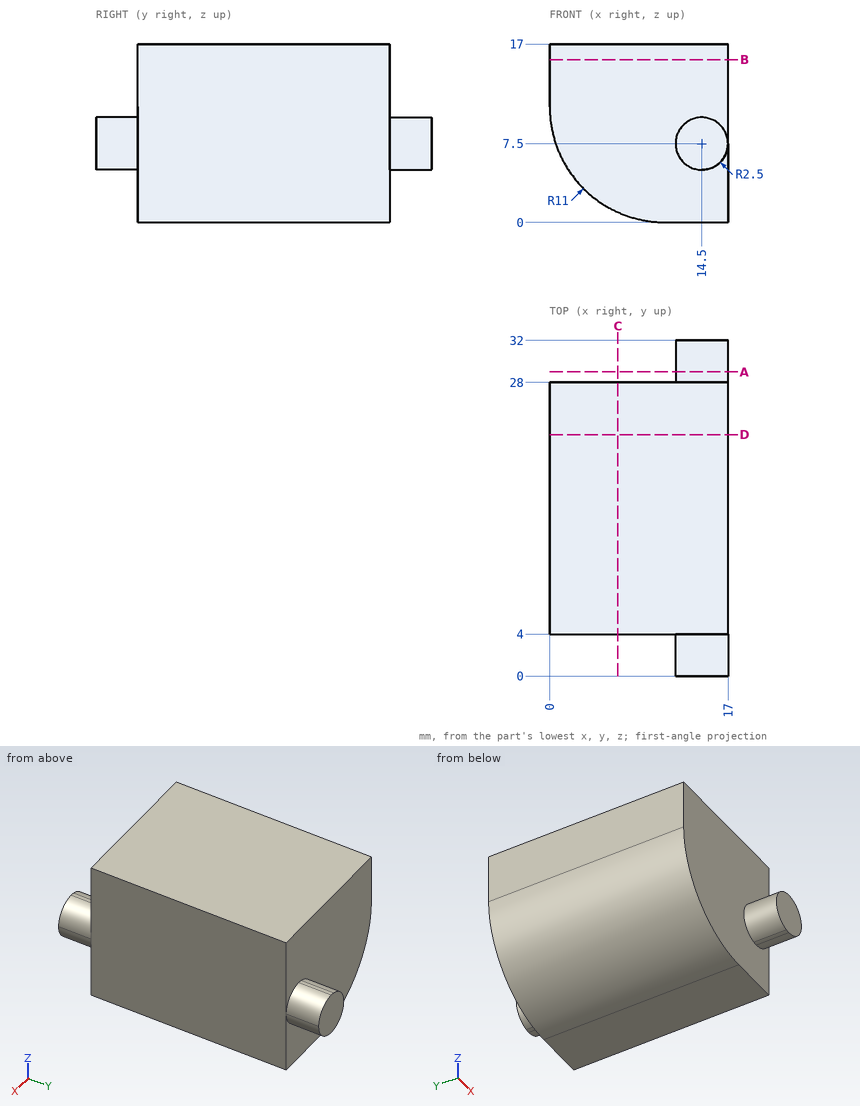
Print and shaded views of the part. All mm, measured from the part's lowest x, y and z. Round coordinates to 2 decimals unless told otherwise and drop trailing zeros. Write each loop counter-clockwise with the first axis right and the second up, starting at its lowest first coordinate (ties: lowest second). Pieces come first, ordered by that corner, then holes.
Item 1: Drop flat-ended pins along their axis: pin 1 Ø2 at (x, z) = (11.5, 12.5) entering from +Y; pin 2 Ø1.5 at (x, z) = (3.5, 12.5) entering from -Y. Give the stop position or say it passes through.
Results:
pin 1: stops at y = 28
pin 2: stops at y = 4
Item 2: Cut at A-A, the plane y = 29. Give the cut face in (x, z).
Results:
outline: circle Ø5 at (14.5, 7.5)
Item 3: Cut at B-B, the plane z = 15.5. Give the cut face in (x, y), plus the area to 3 significant figures.
Results:
outline: (0, 4) - (17, 4) - (17, 28) - (0, 28) - close
area: 408 mm2
Item 4: Probe L1, parallel to Y at x = 8.75, z = 11; L2, parallel to X at y = 9.5, z = 10.75; L3, parallel to Z at x = 1.75, y = 7. List the from-to ranges inside material, lowest first.
Results:
L1: y = 4 to 28
L2: x = 0 to 17
L3: z = 5.05 to 17
Item 5: Cut at C-C, the plane x = 6.5. Give the cut face in (y, z), plus the area to 3 significant figures.
Results:
outline: (4, 0.96) - (28, 0.96) - (28, 17) - (4, 17) - close
area: 385 mm2
Item 6: Cut at D-D, the plane y = 23. Give the cut face in (x, z).
Results:
outline: (0, 11) arc R11 ccw to (11, 0) - (17, 0) - (17, 17) - (0, 17) - close
